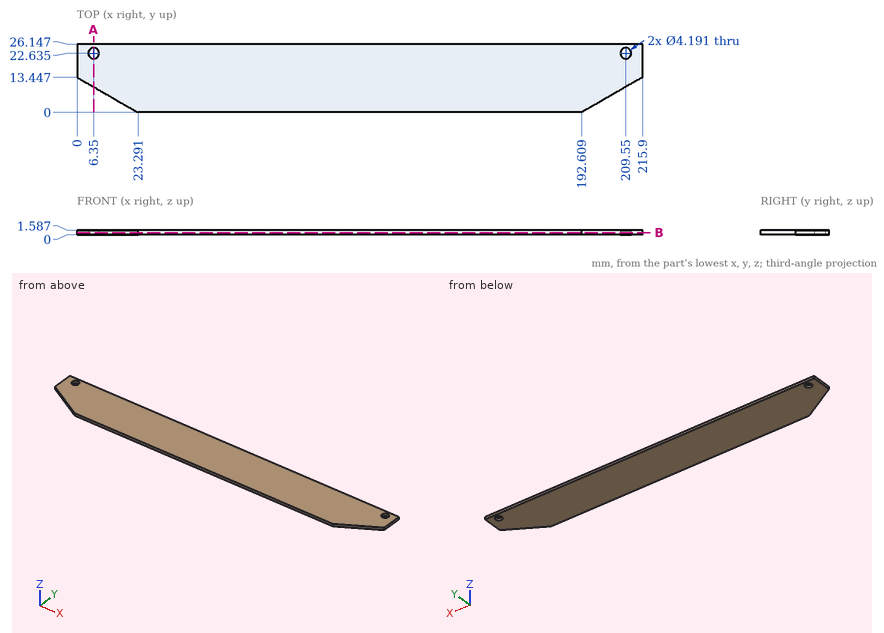
Design review of the part shown in the three views and the two pictorial views. Dimensions are in mm from the part's minimum x, y and z. Coordinates: 2 decimals unless noted, no trailing zeros. Loops run counter-clockwise (first coordinate to the right, second up) from the corner with the lowest first, then second, coordinate; pieces in that order, holes last. Notation, with made-up numbers: M -32.75,14 L 10.25,14 A23 ccw 10.25,43 Z; hole C 26.5,36 d6. An arc over 180 degrees is marked long. Put each result on its own line as item: value. Start each with the question number.
Q1. Wall thickness on line 1 (X direction, y = 22.75, z = 0.35); line 2 (X direction, y = 21.75, z = 1.4); line 3 (Y direction, x = 209.55, z = 0.7) (1 decimal): over which ranges is each line inside the solid? List them lowest first.
Q2. Add section A-A (x = 6.35). Write out the cut boundary in (y, z).
Q3. Clearance check with a flat-ended pin moving along its axis: pin 1 (3.5 mm diameter, centred on x = 6.35, y = 22.64, fed in from +Z). State where the tip first meets the part, or that it passes through.
Q4. Add section B-B (z = 0.8). Count the separate pieces of the cut face and the enclosed holes in it, and give its area (3 significant figures).
Answers:
1. line 1: x = 0 to 4.26, 8.44 to 207.46, 211.64 to 215.9
1. line 2: x = 0 to 4.45, 8.25 to 207.65, 211.45 to 215.9
1. line 3: y = 9.8 to 20.5, 24.7 to 26.1
2. outline: M 9.78,0 L 20.54,0 L 20.54,1.59 L 9.78,1.59 Z; M 24.73,0 L 26.15,0 L 26.15,1.59 L 24.73,1.59 Z
3. pin 1: passes through
4. separate pieces: 1
4. enclosed holes: 2
4. area: 5,300 mm^2
